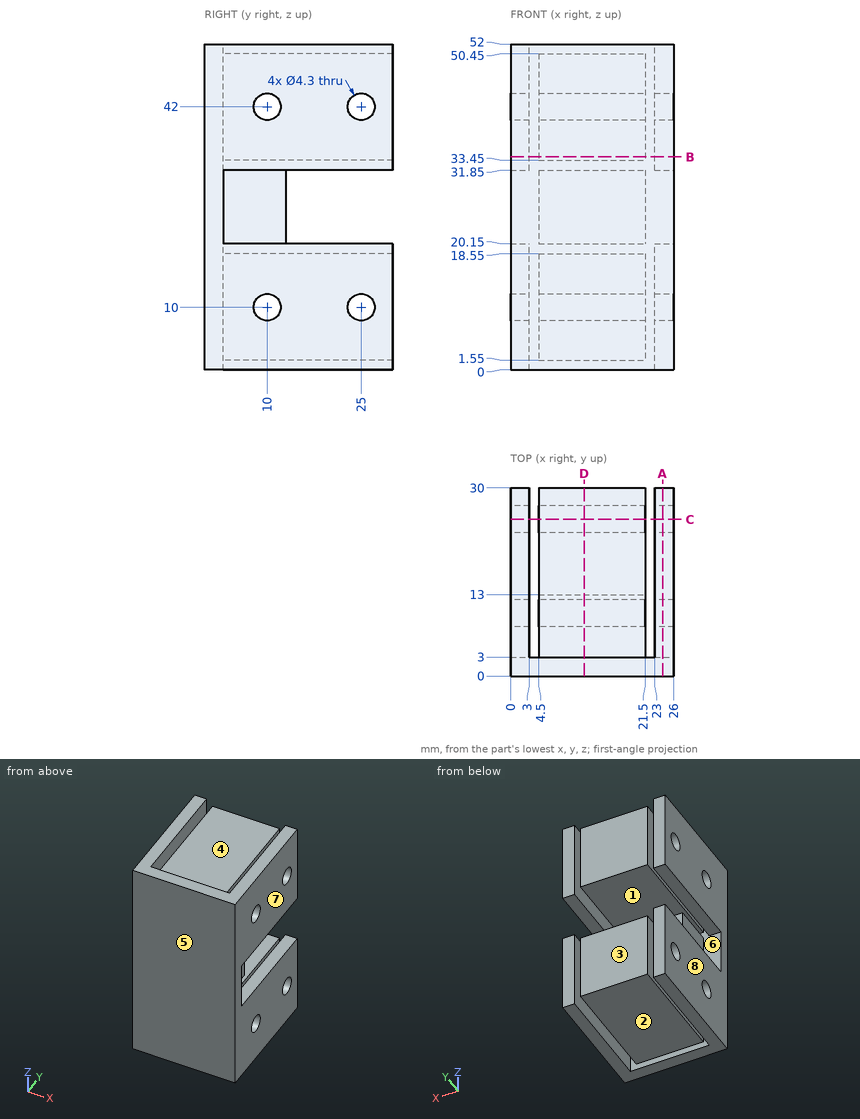
Geometry check sheet. Reference: drawing and pictorial views, mm from the part's lowest x, y, z. A direction names the side the tool comes from. Give positions to 0.01 mm unless a question says otherwise; leave off trailing zeros. Write each loop counter-clockwise with the first axis right and the second up, starting at its lowest first coordinate (ties: lowest second). Pieces come first, ordered by that corner, then holes. Notation, with made-up numbers: (89, 81.5) - (145, 81.5) arc R26 cw to (145, 117.5) - close; hole circle Ø4 at (51, 83.25). An arc over 180 degrees is marked (long way). Use a Markdown table: item, result.
Q1. Section check A-A, the plane x = 24.25. Enter the section's corners in (y, z), then the cut area to 3 significant figures.
Computed:
| item | result |
|---|---|
| outline | (0, 0) - (30, 0) - (30, 20.15) - (3, 20.15) - (3, 31.85) - (30, 31.85) - (30, 52) - (0, 52) - close; hole circle Ø4.3 at (10, 10); hole circle Ø4.3 at (10, 42); hole circle Ø4.3 at (25, 10); hole circle Ø4.3 at (25, 42) |
| area | 1,190 mm² |
Q2. Draft check along X on the marked faces 5, 6, 7 and 8. Enter one of: pulls with the +X half, pulls with the -X half, needs draft (parallel to the pull), parting line crosses it, or undercut.
Computed:
| item | result |
|---|---|
| face 5 | needs draft |
| face 6 | undercut |
| face 7 | pulls with the +X half |
| face 8 | pulls with the -X half |
Q3. Section check B-B, the plane z = 34. Enter the section's corners in (x, y).
Computed:
| item | result |
|---|---|
| outline | (0, 0) - (26, 0) - (26, 30) - (23, 30) - (23, 3) - (21.5, 3) - (21.5, 30) - (4.5, 30) - (4.5, 3) - (3, 3) - (3, 30) - (0, 30) - close |
Q4. Section check C-C, the plane y = 25. Give the number of separate pieces and of enclosed holes in the cut face, then the cut area to 3 significant figures.
Computed:
| item | result |
|---|---|
| separate pieces | 12 |
| enclosed holes | 0 |
| area | 622 mm² |
Q5. Set-up check for the marked faces 1, 2, 3 and 4: record each of +Z, -Z, +X, -X, +Y, -Y from which the full face is reachable in a straight line by a thin tool's end or side.
Computed:
| item | result |
|---|---|
| face 1 | +Y |
| face 2 | -Z, +Y |
| face 3 | +Z, -Z, +X, -X, +Y |
| face 4 | +Z, +Y |
Q6. Go/stop test with flat-tipped pins: P1, Ø2.5, axis at y = 25, z = 42, coming from the +X side; P2, Ø13, axis at x = 11.5, z = 26.5, coming from the +Y side; P3, Ø8.5, axis at x = 12, y = 21.5, coming from the +Z side. Record where each tip stops, or that it passes through.
Computed:
| item | result |
|---|---|
| P1 | passes through |
| P2 | stops at y = 13 |
| P3 | stops at z = 50.45 |
Q7. Thickness scan on L1, parallel to Y at x = 1.5, z = 42; L2, parallel to X at y = 15.5, z = 36.5; L3, parallel to Z at x = 16.75, y = 3.5. Record the ranges inside material, lowest first. Write a range as [from, to].
Computed:
| item | result |
|---|---|
| L1 | y = [0, 7.85], [12.15, 22.85], [27.15, 30] |
| L2 | x = [0, 3], [4.5, 21.5], [23, 26] |
| L3 | z = [1.55, 18.55], [20.15, 31.85], [33.45, 50.45] |
Q8. Section check D-D, the plane x = 11.75. Enter the section's corners in (y, z).
Computed:
| item | result |
|---|---|
| outline | (0, 0) - (3, 0) - (3, 1.55) - (30, 1.55) - (30, 18.55) - (3, 18.55) - (3, 20.15) - (13, 20.15) - (13, 31.85) - (3, 31.85) - (3, 33.45) - (30, 33.45) - (30, 50.45) - (3, 50.45) - (3, 52) - (0, 52) - close; hole circle Ø4.3 at (10, 10); hole circle Ø4.3 at (10, 42); hole circle Ø4.3 at (25, 10); hole circle Ø4.3 at (25, 42) |
